Input: part model. Units: mm. Frame: model coordinates. Face numbers are marked on the shaded views. A direction names the side the tool comes from. Give positions to 0.01 mm unless a question says otherwise; leave off trailing zeros. Loops run counter-clockwise (first coordinate to the right, second up) from the corner with the lowest first, then second, coordinate; pieces in that order, holes last. Notation, with made-up numbers: (-28, 6.25) - (29, 6.25) arc R9 ccw to (29, 19.25) - close; hole circle Ø2 at (3.25, -23.75). An arc over 180 degrees is marked (long way). One line per item, written item: value.
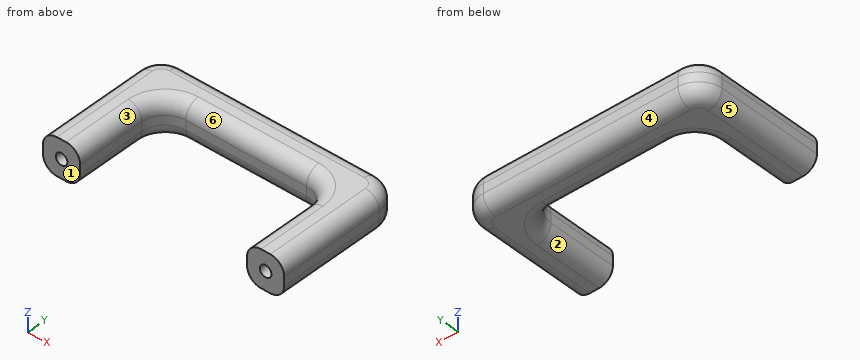
from build123d import *

# Parameters (mm, degrees)
F1_DEPTH = 8
F2_R     = 5
F3_R     = 3
F4_R     = 1.25
F5_DEPTH = 15


with BuildPart() as f1:
    # F0 (on Top) → F1 (new body)
    with BuildSketch(Plane.XY):
        Polygon((44, -30.975605), (-8, -30.975605), (-8, -58.975605), (0, -58.975605), (0, -38.975605), (36, -38.975605), (36, -58.975605), (44, -58.975605), align=None)
    extrude(amount=F1_DEPTH)

    # F2
    f2_edges = [f1.edges().sort_by_distance(p)[0] for p in [
        (-8, -30.975605, 4),
        (44, -30.975605, 4),
        (0, -38.975605, 4),
        (36, -38.975605, 4),
    ]]
    fillet(f2_edges, radius=F2_R)

    # F3
    f3_edges = [f1.edges().sort_by_distance(p)[0] for p in [
        (18, -38.975605, 8),
        (44, -47.475605, 8),
        (44, -47.475605, 0),
        (36, -51.475605, 0),
    ]]
    fillet(f3_edges, radius=F3_R)

    # F4 (on face) → F5 (cut)
    with BuildSketch(Plane.XZ.offset(58.975605)):
        with Locations((40, 4)):
            Circle(F4_R)
        with Locations((-4, 4)):
            Circle(F4_R)
    extrude(amount=-F5_DEPTH, mode=Mode.SUBTRACT)


solid = f1.part
Item 1: Section B-B, the plane x = 16. Output: boundary loops of the cut face in (y, z), and give its area (3 significant figures).
Verdict:
outline: (-38.98, 3) arc R3 ccw to (-35.98, 0) - (-33.98, 0) arc R3 ccw to (-30.98, 3) - (-30.98, 5) arc R3 ccw to (-33.98, 8) - (-35.98, 8) arc R3 ccw to (-38.98, 5) - close
area: 56.3 mm^2
Item 2: Material intervals for L1, parallel to Z at x = 40, y = -48.25; L2, parallel to X at y = -47.5, z = 5; L3, parallel to X at y = -49, z = 6.5, sorted ascending.
Verdict:
L1: z = 0 to 2.75, 5.25 to 8
L2: x = -8 to -4.75, -3.25 to 0, 36 to 39.25, 40.75 to 44
L3: x = -7.6 to -0.4, 36.4 to 43.6
Item 3: Access query for the marked faces 1, 2 and 3. Directions: +Z, -Z, +X, -X, +Y, -Y. A direction counts if a zero-diameter tool reaches every point of the face in a straight line with its end or side. Return the directions, or none.
Verdict:
face 1: +Z, -Z, +X, -X, -Y
face 2: -Z, -Y
face 3: +Z, -Y
Item 4: Draft query along X for the marked faces 4, 5 and 6. Return one class per face: pulls with the +X half, pulls with the -X half, needs draft (parallel to the pull), parting line crosses it, or undercut.
Verdict:
face 4: needs draft
face 5: pulls with the -X half
face 6: undercut
Item 5: Section A-A, the plane y = -46.25. Output: boundary loops of the cut face in (x, z), and give its area (3 significant figures).
Verdict:
outline: (-8, 3) arc R3 ccw to (-5, 0) - (-3, 0) arc R3 ccw to (0, 3) - (0, 5) arc R3 ccw to (-3, 8) - (-5, 8) arc R3 ccw to (-8, 5) - close; (36, 3) arc R3 ccw to (39, 0) - (41, 0) arc R3 ccw to (44, 3) - (44, 5) arc R3 ccw to (41, 8) - (39, 8) arc R3 ccw to (36, 5) - close; hole circle Ø2.5 at (-4, 4); hole circle Ø2.5 at (40, 4)
area: 103 mm^2
Item 6: Section C-C, the plane z = 4. Output: boundary loops of the cut face in (x, y), and give its area (3 significant figures).
Verdict:
outline: (-8, -58.98) - (-5.25, -58.98) - (-5.25, -43.98) - (-2.75, -43.98) - (-2.75, -58.98) - (0, -58.98) - (0, -43.98) arc R5 cw to (5, -38.98) - (31, -38.98) arc R5 cw to (36, -43.98) - (36, -58.98) - (38.75, -58.98) - (38.75, -43.98) - (41.25, -43.98) - (41.25, -58.98) - (44, -58.98) - (44, -35.98) arc R5 ccw to (39, -30.98) - (-3, -30.98) arc R5 ccw to (-8, -35.98) - close
area: 661 mm^2
Item 7: Pin query (flat end, axial travel): P1, Ø1, axis at x = 36.5, y = -45, coming from the +Z side; P2, Ø2, axis at x = 14, z = 3.5, coming from the -Y side; P3, Ø1, axis at x = 0, z = 6, coming from the +Y side. Return the tip coordinate at first contact, or that it passes through.
Verdict:
P1: stops at z = 7.24
P2: stops at y = -38.98
P3: stops at y = -31.02
